Part model, mm, in its own coordinate system. Round coordinates to 2 decimals unless told otherwise and drop trailing zeros. Order: outer loops, then holes, each group sorted by start corner. A loop starts at its lowest first (then second) coordinate and runs counter-clockwise, first axis right, second up. Notation, with made-up numbers: (61, 74) -> (65, 74) arc R18 cw to (65, 80) -> close; hole circle Ø8 at (41.5, 11). An arc over 180 degrees is marked (long way). Answer as a JSON object with one key per item and string values. Group by question number.
```python
from build123d import *

# Parameters (mm, degrees)
SKETCH1_W           = 300
SKETCH1_H           = 420
SKETCH1_R           = 2.5
SKETCH1_R_2         = 1.5
SKETCH1_R_3         = 31.5
BOSS_EXTRUDE1_DEPTH = 8


with BuildPart() as part:
    # Sketch1 → Boss-Extrude1 (new body)
    with BuildSketch(Plane(origin=(0, 0, 0), x_dir=(1, 0, 0), z_dir=(0, 1, 0))):
        Rectangle(SKETCH1_W, SKETCH1_H)
        with Locations(Location((-21, 60, 0), (0, 0, 270))):
            Circle(SKETCH1_R, mode=Mode.SUBTRACT)
        with Locations(Location((21, 60, 0), (0, 0, 90))):
            Circle(SKETCH1_R, mode=Mode.SUBTRACT)
        with Locations(Location((-28.5, -120, 0), (0, 0, 270))):
            Circle(SKETCH1_R_2, mode=Mode.SUBTRACT)
        with Locations(Location((-28.5, -144, 0), (0, 0, 270))):
            Circle(SKETCH1_R_2, mode=Mode.SUBTRACT)
        with Locations(Location((-28.5, -168, 0), (0, 0, 270))):
            Circle(SKETCH1_R_2, mode=Mode.SUBTRACT)
        with Locations(Location((28.5, -168, 0), (0, 0, 90))):
            Circle(SKETCH1_R_2, mode=Mode.SUBTRACT)
        with Locations(Location((28.5, -144, 0), (0, 0, 90))):
            Circle(SKETCH1_R_2, mode=Mode.SUBTRACT)
        with Locations(Location((28.5, -120, 0), (0, 0, 90))):
            Circle(SKETCH1_R_2, mode=Mode.SUBTRACT)
        with Locations(Location((-95, 150, 0), (0, 0, 270))):
            Circle(SKETCH1_R_3, mode=Mode.SUBTRACT)
    extrude(amount=BOSS_EXTRUDE1_DEPTH)


solid = part.part
```
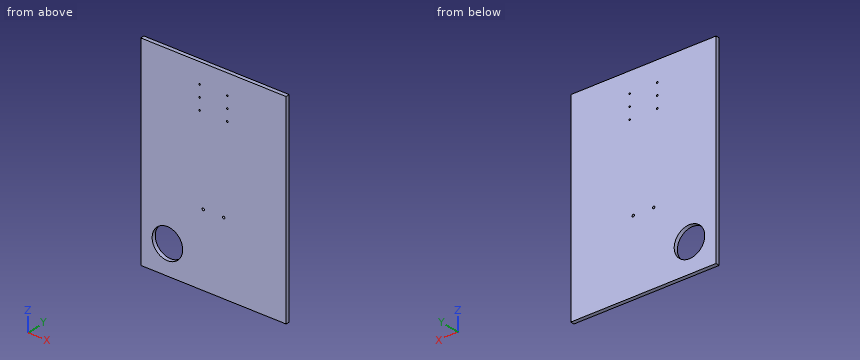
Q1. Band-saw the part on C-C (y = 6.75). Count the separate pieces of the cut face and the enclosed holes in it, plus the area to 3 significant figures.
Q2. Drop a flat-ended pin along its axis: pin 1 Ø3.5 at (x, z) = (28.5, 144) entering from -Y. Give the stop position or say it passes through.
Q3. Wall check: line 1 (X direction, y = 4, z = 119.5); line 2 (Z direction, x = 28.5, y = 5); line 3 (X direction, y = 2.5, z = -150). Give the ranges that are in metal, low to high. Write a range as [from, to].
Q4. Band-saw the part on B-B (z = -150). List the corners of the cut face in (x, y).
Q5. Band-saw the part on A-A (x = -95). List the corners of the cut face in (y, z).
Completed:
{
 "1": {"separate pieces": "1", "enclosed holes": "9", "area": "123,000 mm2"},
 "2": {"pin 1": "y = 0"},
 "3": {"line 1": "[-150, -29.91], [-27.09, 27.09], [29.91, 150]", "line 2": "[-210, 118.5], [121.5, 142.5], [145.5, 166.5], [169.5, 210]", "line 3": "[-150, -126.5], [-63.5, 150]"},
 "4": {"outline": "(-150, 0) -> (-126.5, 0) -> (-126.5, 8) -> (-150, 8) -> close; (-63.5, 0) -> (150, 0) -> (150, 8) -> (-63.5, 8) -> close"},
 "5": {"outline": "(0, -210) -> (8, -210) -> (8, -181.5) -> (0, -181.5) -> close; (0, -118.5) -> (8, -118.5) -> (8, 210) -> (0, 210) -> close"}
}
